```python
from build123d import *

# Parameters (mm, degrees)
F0_W     = 25
F0_H     = 38
F0_W_2   = 20
F0_H_2   = 3
F0_W_3   = 15
F0_H_3   = 25
F1_DEPTH = 1
F2_W     = 22.4918248132
F2_H     = 4.8074135557
F2_W_2   = 20
F2_H_2   = 3
F3_DEPTH = 0.5


with BuildPart() as f1:
    # F0 (on Front) → F1 (new body)
    with BuildSketch(Plane.XZ):
        Rectangle(F0_W, F0_H)
        with Locations((0, -14.5)):
            Rectangle(F0_W_2, F0_H_2, mode=Mode.SUBTRACT)
        with Locations((-1, 2.5)):
            Rectangle(F0_W_3, F0_H_3, mode=Mode.SUBTRACT)
    extrude(amount=F1_DEPTH)

    # F2 (on face) → F3 (join)
    with BuildSketch(Plane(origin=(0, 0, 0), x_dir=(-1, 0, 0), z_dir=(0, 1, 0))):
        with Locations((0.0546504743, -14.3780573271)):
            Rectangle(F2_W, F2_H)
        with Locations((0, -14.5)):
            Rectangle(F2_W_2, F2_H_2, mode=Mode.SUBTRACT)
        with Locations((0, -14.5)):
            Rectangle(F2_W_2, F2_H_2)
    extrude(amount=-F3_DEPTH)


solid = f1.part
```
Here's how the part is built. I have some questions about the finished solid (model axes, mm). A direction names the side the tool comes from. Coordinates: 2 decimals unless noted, no trailing zeros. Order: outer loops, then holes, each group sorted by start corner. A loop starts at its lowest first (then second) coordinate and runs counter-clockwise, first axis right, second up.
1) Imagine slicing it at A-A on x = 1.25. List the corners of the cut face in (y, z) for me, and give its area (3 significant figures).
2) Will these pins go through, and if not, where does the flat tip stop? pin 1 (1 mm diameter, centred on x = 4.5, z = 12.5, fed in from -Y); pin 2 (1.5 mm diameter, centred on x = 0, z = -14, fed in from -Y).
3) Imagine slicing it at C-C on y = -0.65. List the corners of the cut face in (x, z) for me, and give its area (3 significant figures).
4) Imagine slicing it at B-B on z = 12.5. List the corners of the cut face in (x, y) for me.
5) I need wall thicknesses on line 1 (Z direction, x = -4.5, y = -0.75); line 2 (X direction, y = -0.4, z = 14); line 3 (Z direction, x = 1.75, y = -0.4). Which ranges of each line are inside material? Lowest first, please.
6) Which directions (+Z, -Z, +X, -X, +Y, -Y) give clear straight access to the entire face, cutting with the end or side of a thin tool? Please do faces 4 (the face through (-0.2, -0.5, -19)), 5 (the face through (0, -0.5, -14)), 6 (the face through (6.5, -0.5, 2.3)).
7) We'd pull the mould along Y, two halves only. Please class faces 1 (the face through (-0.2, -0.5, 19)), 2 (the face through (-9, 0, 0)), 3 (the face through (-9, -1, 0)): +Y half, -Y half, draft (parallel to the pull), parting line (faces both ways), or undercut.
Response values:
1. outline: (-1, -19) - (0, -19) - (0, -10) - (-1, -10) - (-1, -13) - (-0.5, -13) - (-0.5, -16) - (-1, -16) - close; (-1, 15) - (0, 15) - (0, 19) - (-1, 19) - close
1. area: 11.5 mm2
2. pin 1: passes through
2. pin 2: stops at y = -0.5
3. outline: (-12.5, -19) - (12.5, -19) - (12.5, 19) - (-12.5, 19) - close; hole (-10, -16) - (10, -16) - (10, -13) - (-10, -13) - close; hole (-8.5, -10) - (6.5, -10) - (6.5, 15) - (-8.5, 15) - close
3. area: 515 mm2
4. outline: (-12.5, -1) - (-8.5, -1) - (-8.5, 0) - (-12.5, 0) - close; (6.5, -1) - (12.5, -1) - (12.5, 0) - (6.5, 0) - close
5. line 1: z = -19 to -16, -13 to -10, 15 to 19
5. line 2: x = -12.5 to -8.5, 6.5 to 12.5
5. line 3: z = -19 to -10, 15 to 19
6. face 4: -Z, +X, -X, +Y, -Y
6. face 5: -Y
6. face 6: +Y, -Y
7. face 1: draft
7. face 2: +Y half
7. face 3: -Y half
